Check sheet for the drawn part. Datum: minimum x, y, z corner. Units: mm. A direction names the side the tool comes from. Give positions to 0.01 mm unless a question says otherwise; leave off trailing zeros. Order: outer loops, then holes, each group sorted by start corner. A loop starts at its lowest first (then second) coordinate and runs counter-clockwise, first axis right, second up.
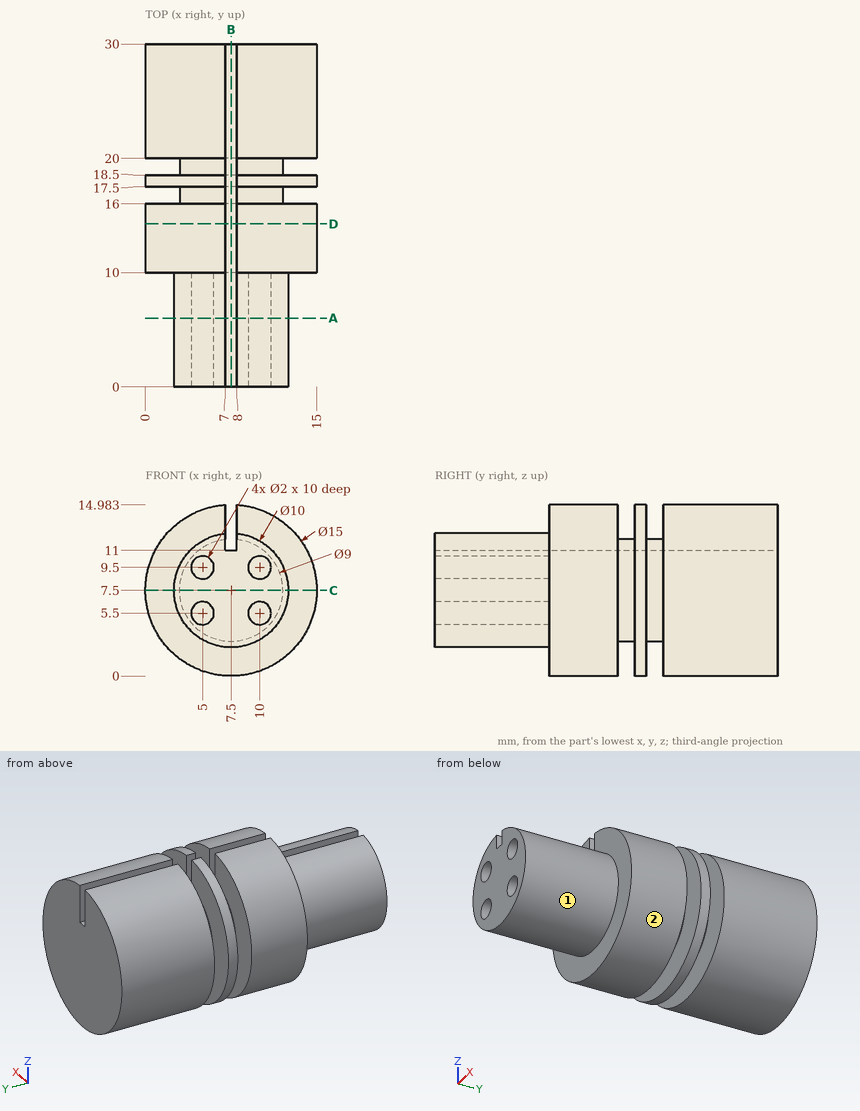
Item 1: Gauge pin test, flat ends, axial feed: pin 1 (1.2 mm diameter, centred on y = 18, z = 13.5, fed in from -X) (1 decimal); pin 2 (4 mm diameter, centred on y = 24, z = 4.5, fed in from +X); pin 3 (1.1 mm diameter, centred on x = 7.5, y = 9.5, fed in from +Z) (3 decimals). Record the tip position at first contact, or that the pin passes through.
Reported:
pin 1: stops at x = 2.3
pin 2: stops at x = 14.93
pin 3: stops at z = 12.475
Item 2: Scan lines: L1, parallel to Y at x = 2.25, z = 7.25; L2, parallel to Z at x = 5, y = 3; L3, parallel to Z at x = 7.25, y = 8.5. Record each from-to range of solid material in increasing order.
Reported:
L1: y = 10 to 16, 17.5 to 18.5, 20 to 30
L2: z = 3.17 to 4.5, 6.5 to 8.5, 10.5 to 11.83
L3: z = 2.51 to 11
Item 3: Sectioned sample at C-C (z = 7.5). Enter the section's corners in (x, y), and give its area (3 significant figures).
Reported:
outline: (0, 10) - (2.5, 10) - (2.5, 0) - (12.5, 0) - (12.5, 10) - (15, 10) - (15, 16) - (12, 16) - (12, 17.5) - (15, 17.5) - (15, 18.5) - (12, 18.5) - (12, 20) - (15, 20) - (15, 30) - (0, 30) - (0, 20) - (3, 20) - (3, 18.5) - (0, 18.5) - (0, 17.5) - (3, 17.5) - (3, 16) - (0, 16) - close
area: 382 mm2
Item 4: Sectioned sample at D-D (y = 14.25). Enter the section's corners in (x, z).
Reported:
outline: (7, 11) - (7, 14.98) arc R7.5 ccw (long way) to (8, 14.98) - (8, 11) - close
Item 5: Set-up check for the marked faces 1 and 2: record each of +Z, -Z, +X, -X, +Y, -Y from which the full face is reachable in a straight line by a thin tool's end or side.
Reported:
face 1: -Y
face 2: +Y, -Y
Item 6: Sectioned sample at A-A (y = 6). Enter the section's corners in (x, z) (1 decimal).
Reported:
outline: (7, 11) - (7, 12.5) arc R5 ccw (long way) to (8, 12.5) - (8, 11) - close; hole circle Ø2 at (5, 5.5); hole circle Ø2 at (5, 9.5); hole circle Ø2 at (10, 5.5); hole circle Ø2 at (10, 9.5)
Item 7: Sectioned sample at B-B (x = 7.5). Enter the section's corners in (y, z), and give its area (3 significant figures).
Reported:
outline: (0, 2.5) - (10, 2.5) - (10, 0) - (16, 0) - (16, 3) - (17.5, 3) - (17.5, 0) - (18.5, 0) - (18.5, 3) - (20, 3) - (20, 0) - (30, 0) - (30, 11) - (0, 11) - close
area: 296 mm2
